Design review of the part built by this model. Coordinates are the model's own, in mm. A direction names the side the tool comes from. Round coordinates to 2 decimals unless told otherwise and drop trailing zeros. Order: outer loops, then holes, each group sorted by start corner. A loop starts at its lowest first (then second) coordinate and runs counter-clockwise, first axis right, second up. Notation, with made-up numbers: (18.25, -6.5) - (54.25, -6.5) arc R19 ccw to (54.25, 1.5) - close; hole circle Ø5 at (4, -34.75). An arc over 180 degrees is marked (long way). Use CSV: the item, a comma, the result in double quotes.
from build123d import *

# Parameters (mm, degrees)
SKETCH2_W           = 203.2
SKETCH2_H           = 127
BOSS_EXTRUDE2_DEPTH = 17.78
FILLET1_R           = 12.7
SKETCH5_R           = 2.0828
CUT_EXTRUDE2_DEPTH  = 12.7
SKETCH6_R           = 2.032
CUT_EXTRUDE3_DEPTH  = 12.7


with BuildPart() as part:
    # Sketch2 → Boss-Extrude2 (new body)
    with BuildSketch(Plane(origin=(0, 0, 0), x_dir=(1, 0, 0), z_dir=(0, 1, 0))):
        Rectangle(SKETCH2_W, SKETCH2_H)
    extrude(amount=BOSS_EXTRUDE2_DEPTH)

    # Fillet1
    fillet1_edges = [part.edges().sort_by_distance(p)[0] for p in [
        (-101.6, 8.89, -63.5),
        (101.6, 8.89, -63.5),
    ]]
    fillet(fillet1_edges, radius=FILLET1_R)

    # Sketch5 → Cut-Extrude2 (cut)
    with BuildSketch(Plane.XZ):
        with Locations((50.8, 49.8348)):
            Circle(SKETCH5_R)
        with Locations((33.5788, 25.0698)):
            Circle(SKETCH5_R)
        with Locations((-50.8, 25.0698)):
            Circle(SKETCH5_R)
        with Locations((-33.5788, 49.8348)):
            Circle(SKETCH5_R)
    extrude(amount=-CUT_EXTRUDE2_DEPTH, mode=Mode.SUBTRACT)

    # Sketch6 → Cut-Extrude3 (cut)
    with BuildSketch(Plane(origin=(0, 17.78, 0), x_dir=(1, 0, 0), z_dir=(0, 1, 0))):
        with Locations((-8.13412282, 25.4)):
            Circle(SKETCH6_R)
        with Locations((50.8, 1.756413821)):
            Circle(SKETCH6_R)
        with Locations((-21.251584432, -7.296651341)):
            Circle(SKETCH6_R)
        with Locations((37.682538388, -30.94023752)):
            Circle(SKETCH6_R)
    extrude(amount=-CUT_EXTRUDE3_DEPTH, mode=Mode.SUBTRACT)


solid = part.part
1) To check wall thickness, follow L1, parallel to X at y = 7.5, z = 50; L2, parallel to X at y = 9.75, z = -2; L3, parallel to X at y = 14.75, z = 8. State the ranges of each line that lie inside material, in increasing order. Write a range as from..to.
Data:
L1,"x = -101.6..-35.66, -31.5..48.72, 52.88..101.6"
L2,"x = -101.6..48.78, 52.82..101.6"
L3,"x = -101.6..-23.16, -19.35..101.6"
2) For faces 1 (the face through (-32.618, 6.261, 47.987)), 2 (the face through (97.98, 9.01, -59.68)), 3 (the face through (51, 5.08, -2)), list the 3-axis set-ups (+Z, -Z, +X, -X, +Y, -Y) from which the entire face can be reached by the end or side of a thin tool; tool diameter is ignored.
Data:
face 1,"-Y"
face 2,"-Z, +X, +Y, -Y"
face 3,"+Y"
3) We need section B-B (x = -50.8). Give the boundary of the cut face in (y, z), then the cut area to 3 significant figures.
Data:
outline,"(0, -63.5) - (17.78, -63.5) - (17.78, 63.5) - (0, 63.5) - (0, 27.15) - (12.7, 27.15) - (12.7, 22.99) - (0, 22.99) - close"
area,"2,210 mm2"
4) We need section A-A (x = 50.8). Give the boundary of the cut face in (y, z).
Data:
outline,"(0, -63.5) - (17.78, -63.5) - (17.78, -3.79) - (5.08, -3.79) - (5.08, 0.28) - (17.78, 0.28) - (17.78, 63.5) - (0, 63.5) - (0, 51.92) - (12.7, 51.92) - (12.7, 47.75) - (0, 47.75) - close"
5) Insertion check: pin 1 Ø3.5 at (x, z) = (-50.8, 25.07) entering from -Y; pin 2 Ø1.2 at (x, z) = (51.5, -1.5) entering from +Y. Each pin has a flat end and moves straight along its axis. Give the tip position at first contact, or say it passes through.
Data:
pin 1,"stops at y = 12.7"
pin 2,"stops at y = 5.08"
6) The part is to be moulded in two halves that separate along X. For faces 4 (the face through (-97.98, 9.01, -59.68)), 5 (the face through (-1, 9, -63.5)), 6 (the face through (38, 5.08, 31)), 7 (the face through (-49.68, 6.261, 26.826)), say which applies: +X half, -X half, draft (parallel to the pull), parting line (faces both ways), or undercut.
Data:
face 4,"-X half"
face 5,"draft"
face 6,"undercut"
face 7,"undercut"
